Part print with two shaded views. Sizes in mm from the minimum x, y, z corner. A direction names the side the tool comes from. Give positions to 0.01 mm unless a question says otherwise; leave off trailing zeros. Loops run counter-clockwise (first coordinate to the right, second up) from the corner with the lowest first, then second, coordinate; pieces in that order, holes last. Notation, with made-up numbers: M -19,54.25 L 33,54.25 A18 ccw 33,81.25 Z; hole C -6.5,19.25 d9. An arc over 180 degrees is marked long. Answer as a JSON object with one key per item and string values. Group by question number.
1. Slice it at D-D (y = 10). List the corners of the cut face in (x, z), then the cut area to 3 significant figures.
2. Slice it at B-B (x = 12). List the corners of the cut face in (y, z) (1 decimal).
3. Drop flat-ended pins along their axis: pin 1 Ø4 at (x, z) = (5.5, 11.5) entering from -Y; pin 2 Ø1.6 at (y, z) = (7.5, 1) entering from +X; pin 3 Ø1 at (x, z) = (4, 1.5) entering from +Y. Give the stop position or say it passes through.
4. 3-axis set-ups, long thin cutter, end or side, ignore diameter. For the marked faces 1, 2 and 3: which of +Z, -Z, +X, -X, +Y, -Y reach the whole face in a straight line?
5. Slice it at C-C (z = 19). List the corners of the cut face in (x, y).
6. Slice it at A-A (y = 5.5). List the corners of the cut face in (x, z).
7. Drill centre lines: line 1 along Z through (x, y) = (9.5, 10.25); line 2 along Z through (x, y) = (4.75, 4.25); line 3 along X through (y, z) = (8.25, 1). Where is each one in solid material? Low to high. Write a range as [from, to].
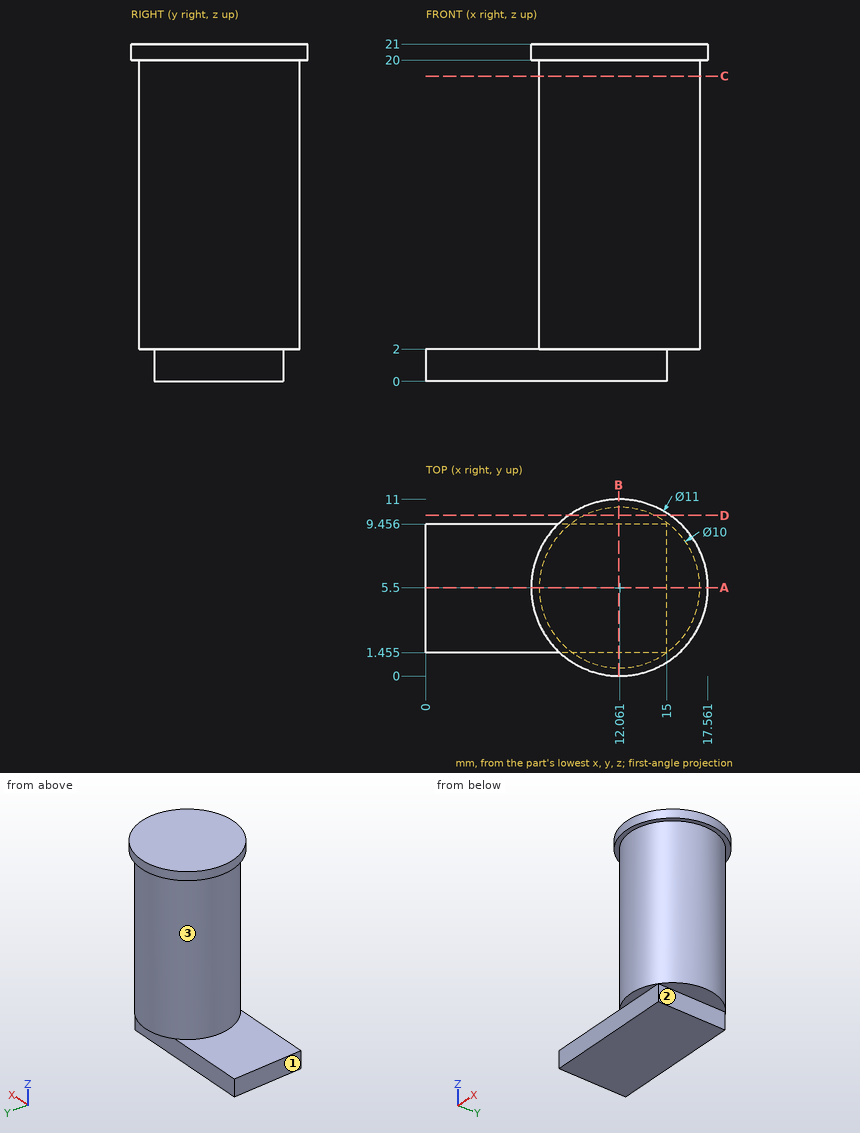
Established:
{
 "1": {"outline": "M 8.9,20 L 9.88,20 L 9.88,2 L 14.24,2 L 14.24,20 L 15.22,20 L 15.22,21 L 8.9,21 Z", "area": "84.8 mm^2"},
 "2": {"outline": "M 0,20 L 0.5,20 L 0.5,2 L 1.5,2 L 1.5,0 L 9.5,0 L 9.5,2 L 10.5,2 L 10.5,20 L 11,20 L 11,21 L 0,21 Z"},
 "3": {"pin 1": "stops at y = 3.45", "pin 2": "stops at x = 15", "pin 3": "stops at y = 9.46"},
 "4": {"face 1": "+Z, -Z, -X, +Y, -Y", "face 2": "-Z, +X, +Y, -Y", "face 3": "none"},
 "5": {"outline": "C 12.06,5.5 d10"},
 "6": {"outline": "M 0,0 L 15,0 L 15,2 L 17.06,2 L 17.06,20 L 17.56,20 L 17.56,21 L 6.56,21 L 6.56,20 L 7.06,20 L 7.06,2 L 0,2 Z"},
 "7": {"line 1": "z = [20, 21]", "line 2": "z = [0, 2]", "line 3": "x = [0, 15]"}
}
